Check sheet for the modelled part. Datum: model origin and axes. Units: mm. A direction names the side the tool comes from. Round coordinates to 2 decimals unless told otherwise and drop trailing zeros. Order: outer loops, then holes, each group sorted by start corner. A loop starts at its lowest first (then second) coordinate and runs counter-clockwise, first axis right, second up. Notation, with made-up numbers: M 87.25,-40 L 92.25,-40 A12 cw 92.25,-29 Z; hole C -19,77.5 d4. An arc over 180 degrees is marked long. One line per item, written item: value. Start each with the question number.
(1) Thickness scan on L1, parallel to Y at x = 205, z = -56; L2, parallel to Z at x = 198, y = 41; L3, parallel to Y at x = 169, z = 5. Record the ranges inside material, lowest first.
(2) Cross-section at C-C, the plane y = -16. Enter the section's corners in (x, z), and give its area (3 significant figures).
(3) Depth check by flat-ended pin: pin 1 Ø7.5 at (x, z) = (59, 19) entering from +Y; pin 2 Ø4.5 at (x, z) = (64.5, 2) entering from -Y; pin 3 Ø24 at (y, z) = (18.5, 2.5) entering from -X; pin 4 Ø16.5 at (x, y) = (63, -2) entering from +Z. Enter the tip coordinate at first touch or a pass-through.
(4) Cross-section at B-B, the plane y = 73. Enter the section's corners in (x, z), and give its area (4 significant figures).
(5) Cross-section at A-A, the plane x = 205. Enter the section's corners in (y, z).
(6) Access from +Z, -Z, +X, -X, +Y, -Y to the whole of each face (thin tool, end or side, straight path). Record for faces 1 (the face through (70, 29, 0)), 2 (the face through (190, 64, -53)), 3 (the face through (62, 24, 16)).
(7) Cross-section at D-D, the plane z = -3. Enter the section's corners in (x, y), and give its area (3 significant figures).
(8) Release check for a two-part mould opening along Z. For faces 4 (the face through (205, 40, 52.5)), 5 (the face through (97, 111, 7.5)), 6 (the face through (199.505, -15.758, -59.895)), 7 (the face through (205, 40, -52.5)) record: released by +Z, released by -Z, zero draft, split by the parting line, or undercut.
from build123d import *

# Parameters (mm, degrees)
SKETCH1_R                = 12
BOSS_EXTRUDE1_DEPTH      = 55
SKETCH4_W                = 48
SKETCH4_H                = 48
BOSS_EXTRUDE3_DEPTH      = 15
SKETCH5_W                = 15
SKETCH5_H                = 15
BOSS_EXTRUDE4_DEPTH      = 100
SKETCH6_W                = 15
SKETCH6_H                = 15
BOSS_EXTRUDE6_DEPTH      = 150
BOSS_EXTRUDE7_DEPTH      = 60
BOSS_EXTRUDE7_DEPTH_BACK = 75
SKETCH7_W                = 30
SKETCH7_H                = 15
SKETCH8_W                = 30
SKETCH8_H                = 15
BOSS_EXTRUDE8_DEPTH      = 140
SKETCH9_R                = 5.5
CUT_EXTRUDE1_DEPTH       = 287.358167336


with BuildPart() as part:
    # Sketch1 → Boss-Extrude1 (new body)
    with BuildSketch(Plane(origin=(0, 0, 0), x_dir=(0, 0, -1), z_dir=(1, 0, 0))):
        Circle(SKETCH1_R)
    extrude(amount=BOSS_EXTRUDE1_DEPTH)

    # Sketch4 → Boss-Extrude3 (add)
    with BuildSketch(Plane(origin=(55, 0, 0), x_dir=(0, 0, -1), z_dir=(1, 0, 0))):
        Rectangle(SKETCH4_W, SKETCH4_H)
    extrude(amount=BOSS_EXTRUDE3_DEPTH)

    # Sketch5 → Boss-Extrude4 (add)
    with BuildSketch(Plane(origin=(0, 24, 0), x_dir=(1, 0, 0), z_dir=(0, 1, 0))):
        with Locations((62.5, 0)):
            Rectangle(SKETCH5_W, SKETCH5_H)
    extrude(amount=BOSS_EXTRUDE4_DEPTH)

    # Sketch6 → Boss-Extrude6 (add)
    with BuildSketch(Plane(origin=(70, 0, 0), x_dir=(0, 0, -1), z_dir=(1, 0, 0))):
        with Locations((0, 116.5)):
            Rectangle(SKETCH6_W, SKETCH6_H)
    extrude(amount=BOSS_EXTRUDE6_DEPTH)

    # Sketch7 → Boss-Extrude7 (add, two sides: drawn at the far end of the back side and taken through both)
    with BuildSketch(Plane(origin=(0, 0, -7.5), x_dir=(-1, 0, 0), z_dir=(0, 0, -1)).offset(-BOSS_EXTRUDE7_DEPTH_BACK)):
        with Locations((-205, 116.5)):
            Rectangle(SKETCH7_W, SKETCH7_H)
    extrude(amount=BOSS_EXTRUDE7_DEPTH + BOSS_EXTRUDE7_DEPTH_BACK)

    # Sketch8 → Boss-Extrude8 (add)
    with BuildSketch(Plane.XZ.offset(-109)):
        with Locations((205, -60)):
            Rectangle(SKETCH8_W, SKETCH8_H)
        with Locations((205, 60)):
            Rectangle(SKETCH8_W, SKETCH8_H)
    extrude(amount=BOSS_EXTRUDE8_DEPTH)

    # Sketch9 → Cut-Extrude1 (cut, through all)
    with BuildSketch(Plane.XY.offset(67.5)):
        with Locations((205, -16)):
            Circle(SKETCH9_R)
    extrude(amount=-CUT_EXTRUDE1_DEPTH, mode=Mode.SUBTRACT)


solid = part.part
Values found:
1. L1: -31 to -21.5, -10.5 to 124
1. L2: -67.5 to -52.5, 52.5 to 67.5
1. L3: 109 to 124
2. outline: M 55,-24 L 70,-24 L 70,24 L 55,24 Z; M 190,-67.5 L 199.5,-67.5 L 199.5,-52.5 L 190,-52.5 Z; M 190,52.5 L 199.5,52.5 L 199.5,67.5 L 190,67.5 Z; M 210.5,-67.5 L 220,-67.5 L 220,-52.5 L 210.5,-52.5 Z; M 210.5,52.5 L 220,52.5 L 220,67.5 L 210.5,67.5 Z
2. area: 1,290 mm^2
3. pin 1: y = 24
3. pin 2: y = -24
3. pin 3: x = 0
3. pin 4: z = 24
4. outline: M 55,-7.5 L 70,-7.5 L 70,7.5 L 55,7.5 Z; M 190,-67.5 L 220,-67.5 L 220,-52.5 L 190,-52.5 Z; M 190,52.5 L 220,52.5 L 220,67.5 L 190,67.5 Z
4. area: 1,125 mm^2
5. outline: M -31,-67.5 L -21.5,-67.5 L -21.5,-52.5 L -31,-52.5 Z; M -31,52.5 L -21.5,52.5 L -21.5,67.5 L -31,67.5 Z; M -10.5,-67.5 L 124,-67.5 L 124,67.5 L -10.5,67.5 L -10.5,52.5 L 109,52.5 L 109,-52.5 L -10.5,-52.5 Z
6. face 1: +Z, -Z, +X, -Y
6. face 2: -Z, -X, +Y, -Y
6. face 3: +Z, +X, -X, +Y
7. outline: M 0,-11.62 L 55,-11.62 L 55,-24 L 70,-24 L 70,109 L 220,109 L 220,124 L 55,124 L 55,11.62 L 0,11.62 Z
7. area: 5,750 mm^2
8. face 4: undercut
8. face 5: released by +Z
8. face 6: zero draft
8. face 7: undercut
